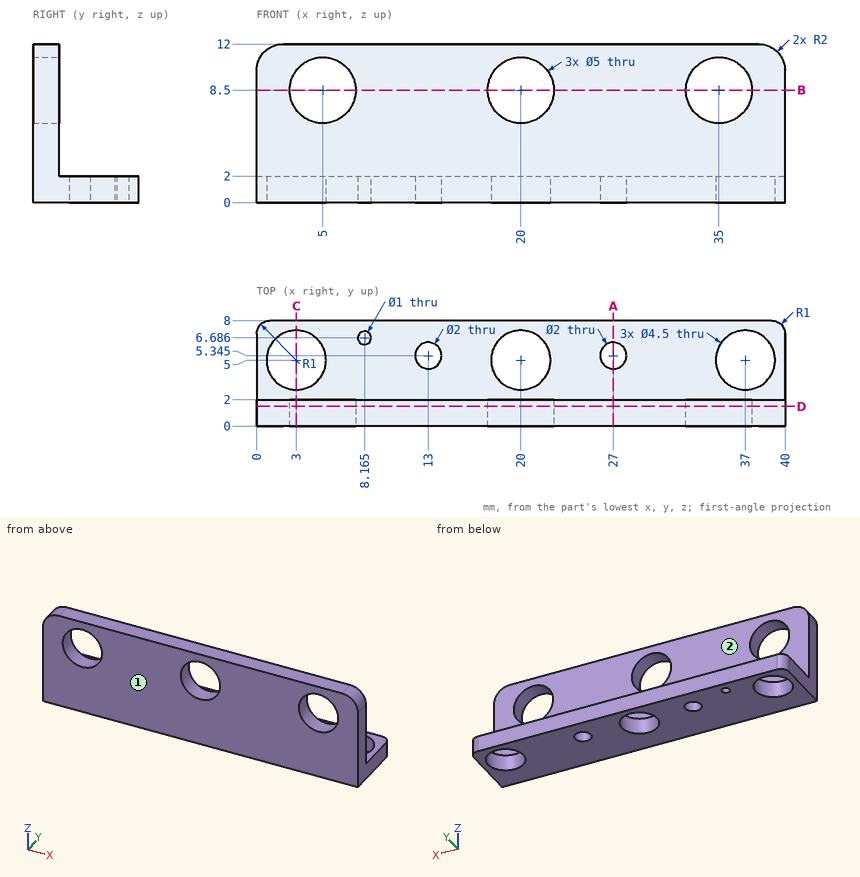
Job drawing, mm, ordinate dimensions from the low corner. One solid piece. A direction names the side the tool comes from. Give positions to 0.01 mm unless a question says otherwise; leave off trailing zeros. Write each loop counter-clockwise with the first axis right and the second up, starting at its lowest first coordinate (ties: lowest second). Pieces come first, ordered by that corner, then holes. Notation, with made-up numbers: M -22.5,61 L -18.5,61 A32 ccw -18.5,99 Z; hole C -7.75,-26 d5. An arc over 180 degrees is marked long. One line per item, written item: value. Start each with the question number.
Q1. Saw through at D-D, the plane y = 1.5. Write the cut outline in (x, z).
Q2. Saw through at A-A, the plane x = 27. Write the cut outline in (y, z) (1 decimal).
Q3. Drop flat-ended pins along their axis: pin 1 Ø6 at (x, z) = (9, 4.5) entering from -Y; pin 2 Ø3 at (x, y) = (16.5, 5) entering from +Z; pin 3 Ø2.5 at (x, y) = (3, 5) entering from -Z (3 decimals); pin 4 Ø5 at (x, z) = (13, 5.5) entering from +Y. Give the stop position or say it passes through.
Q4. Saw through at B-B, the plane z = 8.5. Write the cut outline in (x, y).
Q5. Probe probe 1 along X at (y, z) = (0.8, 8.5); probe 2 along Y at (x, z) = (37, 1.3); probe 3 along Y at (x, z) = (27, 1.65) (1 decimal). List the from-to ranges inside material, lowest first. Write a range as [from, to].
Q6. Saw through at C-C, the plane x = 3. Write the cut outline in (y, z).
Q7. 3-axis set-ups, long thin cutter, end or side, ignore diameter. For the marked faces 1 and 2: which of +Z, -Z, +X, -X, +Y, -Y reach the whole face in a straight line?
Output values:
1. outline: M 0,0 L 40,0 L 40,10 A2 ccw 38,12 L 2,12 A2 ccw 0,10 Z; hole C 5,8.5 d5; hole C 20,8.5 d5; hole C 35,8.5 d5
2. outline: M 0,0 L 4.3,0 L 4.3,2 L 2,2 L 2,12 L 0,12 Z; M 6.3,0 L 8,0 L 8,2 L 6.3,2 Z
3. pin 1: stops at y = 0
3. pin 2: stops at z = 2
3. pin 3: passes through
3. pin 4: stops at y = 2
4. outline: M 0,0 L 2.5,0 L 2.5,2 L 0,2 Z; M 7.5,0 L 17.5,0 L 17.5,2 L 7.5,2 Z; M 22.5,0 L 32.5,0 L 32.5,2 L 22.5,2 Z; M 37.5,0 L 40,0 L 40,2 L 37.5,2 Z
5. probe 1: x = [0, 2.5], [7.5, 17.5], [22.5, 32.5], [37.5, 40]
5. probe 2: y = [0, 2.75], [7.25, 8]
5. probe 3: y = [0, 4.3], [6.3, 8]
6. outline: M 0,0 L 2.75,0 L 2.75,2 L 2,2 L 2,7 L 0,7 Z; M 0,10 L 2,10 L 2,12 L 0,12 Z; M 7.25,0 L 8,0 L 8,2 L 7.25,2 Z
7. face 1: +Z, -Z, +X, -X, -Y
7. face 2: +Z, +X, -X, +Y
